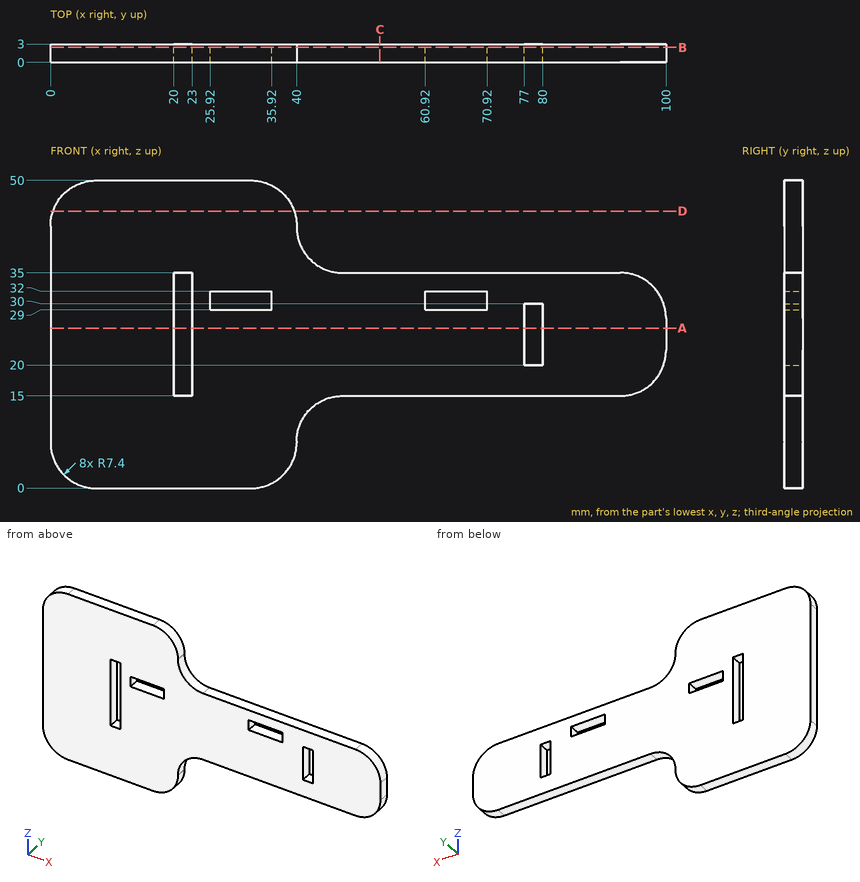
Design review of the part shown in the three views and the two pictorial views. Dimensions are in mm from the part's minimum x, y and z. Round coordinates to 2 decimals unless told otherwise and drop trailing zeros. Loops run counter-clockwise (first coordinate to the right, second up) from the corner with the lowest first, then second, coordinate; pieces in that order, holes last. Notation, with made-up numbers: (11.25, 62.25) - (57.25, 62.25) arc R24 ccw to (57.25, 85.25) - close; hole circle Ø5 at (-22.5, 30). An arc over 180 degrees is marked (long way). Use one line per item in the form item = value.
1) We need section C-C on x = 53.5. Write out the cut boundary in (y, z), then the cut area to 3 significant figures.
Solutions:
outline = (0, 15) - (3, 15) - (3, 35) - (0, 35) - close
area = 60.0 mm2
2) We need section B-B on y = 2.45. State how many separate pieces and enclosed holes the cut face has, then the cut area to 3 significant figures.
Solutions:
separate_pieces = 1
enclosed_holes = 4
area = 3,000 mm2
3) We need section D-D on z = 45. Write out the cut boundary in (x, y).
Solutions:
outline = (0.4, 0) - (39.6, 0) - (39.6, 3) - (0.4, 3) - close
4) Wall thickness on probe 1 along X at (y, z) = (2, 27.5); probe 2 along Z at (x, y) = (67, 0.65); probe 3 along X at (y, z) = (2, 30.5): over which ranges is each line inside the solid? List them lowest first.
Solutions:
probe_1 = 0 to 20, 23 to 77, 80 to 100
probe_2 = 15 to 29, 32 to 35
probe_3 = 0 to 20, 23 to 25.92, 35.92 to 60.92, 70.92 to 99.41
5) Clearance check with flat-ended pins moving along their axes: P1, Ø0.9, axis at y = 1.5, z = 30, coming from the +X side; P2, Ø1, axis at y = 2.5, z = 44.5, coming from the +X side; P3, Ø0.9, axis at x = 79, y = 1, coming from the +Z side; P4, Ø4, axis at x = 85.5, z = 37.5, coming from the +Y side. State where each tip first meets the part, or that it passes through.
Solutions:
P1 = 99.74
P2 = 39.87
P3 = 35
P4 = through
6) We need section A-A on z = 26. Write out the cut boundary in (x, y).
Solutions:
outline = (0, 0) - (20, 0) - (20, 3) - (0, 3) - close; (23, 0) - (77, 0) - (77, 3) - (23, 3) - close; (80, 0) - (100, 0) - (100, 3) - (80, 3) - close
